from build123d import *

# Parameters (mm, degrees)
SKETCH1_W           = 6.2
SKETCH1_H           = 6.2
BOSS_EXTRUDE1_DEPTH = 90
SKETCH2_W           = 6.2
SKETCH2_H           = 3
SKETCH2_R           = 2.2
CUT_EXTRUDE1_DEPTH  = 10


with BuildPart() as part:
    # Sketch1 → Boss-Extrude1 (new body)
    with BuildSketch(Plane.XY):
        Rectangle(SKETCH1_W, SKETCH1_H)
    extrude(amount=BOSS_EXTRUDE1_DEPTH)

    # Sketch2 → Cut-Extrude1 (cut)
    with BuildSketch(Plane(origin=(0, 3.1, 0), x_dir=(1, 0, 0), z_dir=(0, 1, 0))):
        with Locations((0, -1.5)):
            Rectangle(SKETCH2_W, SKETCH2_H)
        with Locations(Location((0, -7.5, 0), (0, 0, 270))):
            Circle(SKETCH2_R)
    extrude(amount=-CUT_EXTRUDE1_DEPTH, mode=Mode.SUBTRACT)


solid = part.part
Geometry: final body of the model. Coordinates: model frame, mm. Give positions to 0.01 mm unless a question says otherwise; leave off trailing zeros. Order: outer loops, then holes, each group sorted by start corner. A loop starts at its lowest first (then second) coordinate and runs counter-clockwise, first axis right, second up. Notation, with made-up numbers: (-6.75, -30.75) -> (8.25, -30.75) arc R33 cw to (8.25, 2.25) -> close; hole circle Ø6 at (-17.5, 35). An arc over 180 degrees is marked (long way). Answer as a JSON object with one key per item and string values.
Q1. Material intervals for probe 1 along Z at (x, y) = (-0.25, 0.25); probe 2 along X at (y, z) = (0.75, 7.5); probe 3 along Z at (x, y) = (-0.5, 0), sorted ascending.
Entries:
{"probe 1": "z = 3 to 5.31, 9.69 to 90", "probe 2": "x = -3.1 to -2.2, 2.2 to 3.1", "probe 3": "z = 3 to 5.36, 9.64 to 90"}
Q2. Draft query along X for faces 1 (the cylindrical face through (-0.843, 0.043, 9.532)), 2 (the flat face through (-3.1, 0, 46)), 3 (the flat face through (0, 0, 90)). Return one class per face: released by +X, released by -X, zero draft, split by the parting line, or undercut.
Entries:
{"face 1": "undercut", "face 2": "released by -X", "face 3": "zero draft"}
Q3. Section C-C (y = 1.25). Output: boundary loops of the cut face in (x, z).
Entries:
{"outline": "(-3.1, 3) -> (3.1, 3) -> (3.1, 90) -> (-3.1, 90) -> close; hole circle Ø4.4 at (0, 7.5)"}
Q4. Section A-A (z = 7.5). Output: boundary loops of the cut face in (x, y), plus the area to 3 significant figures.
Entries:
{"outline": "(-3.1, -3.1) -> (-2.2, -3.1) -> (-2.2, 3.1) -> (-3.1, 3.1) -> close; (2.2, -3.1) -> (3.1, -3.1) -> (3.1, 3.1) -> (2.2, 3.1) -> close", "area": "11.2 mm^2"}
Q5. Section B-B (x = 0). Output: boundary loops of the cut face in (y, z).
Entries:
{"outline": "(-3.1, 3) -> (3.1, 3) -> (3.1, 5.3) -> (-3.1, 5.3) -> close; (-3.1, 9.7) -> (3.1, 9.7) -> (3.1, 90) -> (-3.1, 90) -> close"}
